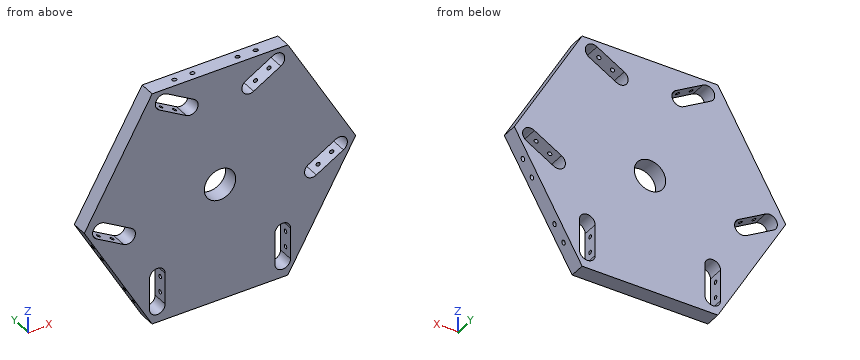
```python
from build123d import *

# Parameters (mm, degrees)
BOSS_EXTRUDE1_DEPTH     = 10
CUT_EXTRUDE1_DEPTH      = 20
SKETCH4_R               = 1.25
CUT_EXTRUDE2_DEPTH      = 149.417392118
CUT_EXTRUDE3_DEPTH      = 116
CUT_EXTRUDE3_DEPTH_BACK = 116
SKETCH6_R               = 10
CIRPATTERN1_COUNT       = 3


with BuildPart() as part:
    # Sketch1 → Boss-Extrude1 (new body)
    with BuildSketch(Plane(origin=(0, 0, 0), x_dir=(1, 0, 0), z_dir=(0, 1, 0))):
        Polygon((-43.301270189, -75), (43.301270189, -75), (86.602540378, 0), (43.301270189, 75), (-43.301270189, 75), (-86.602540378, 0), align=None)
    extrude(amount=BOSS_EXTRUDE1_DEPTH)

    # Sketch3 → Cut-Extrude1 (cut)
    with BuildSketch(Plane(origin=(0, 10, 0), x_dir=(1, 0, 0), z_dir=(0, 1, 0))):
        with BuildLine():
            Line((-78.791651246, 6.47114317), (-61.47114317, 16.47114317))
            ThreePointArc((-61.47114317, 16.47114317), (-54.641016151, 14.641016151), (-56.47114317, 7.810889132))
            Line((-56.47114317, 7.810889132), (-73.791651246, -2.189110868))
            ThreePointArc((-73.791651246, -2.189110868), (-80.621778265, -0.358983849), (-78.791651246, 6.47114317))
        make_face()
        with BuildLine():
            Line((-38.791651246, -62.810889132), (-21.47114317, -52.810889132))
            ThreePointArc((-21.47114317, -52.810889132), (-14.641016151, -54.641016151), (-16.47114317, -61.47114317))
            Line((-16.47114317, -61.47114317), (-33.791651246, -71.47114317))
            ThreePointArc((-33.791651246, -71.47114317), (-40.621778265, -69.641016151), (-38.791651246, -62.810889132))
        make_face()
    cut_extrude1 = extrude(amount=-CUT_EXTRUDE1_DEPTH, mode=Mode.SUBTRACT)

    # Sketch4 → Cut-Extrude2 (cut, symmetric)
    with BuildSketch(Plane(origin=(17.5, 0, 30.310889132), x_dir=(0.8660254037844383, 0, -0.5000000000000007), z_dir=(0.5000000000000007, 0, 0.8660254037844383))):
        with Locations((-60, 5)):
            Circle(SKETCH4_R)
        with Locations((-50, 5)):
            Circle(SKETCH4_R)
    cut_extrude2 = extrude(amount=CUT_EXTRUDE2_DEPTH, both=True, mode=Mode.SUBTRACT)

    # Sketch6 → Cut-Extrude3 (cut, two sides: drawn at the far end of the back side and taken through both)
    with BuildSketch(Plane(origin=(0, 10, 0), x_dir=(1, 0, 0), z_dir=(0, 1, 0)).offset(-CUT_EXTRUDE3_DEPTH_BACK)):
        with Locations(Location((0, 0, 0), (0, 0, 270))):
            Circle(SKETCH6_R)
    extrude(amount=CUT_EXTRUDE3_DEPTH + CUT_EXTRUDE3_DEPTH_BACK, mode=Mode.SUBTRACT)

    # CirPattern1: Cut-Extrude1, Cut-Extrude2 ×3 about axis
    cirpattern1_axis = Axis((0, 0, 0), (0, 1, 0))
    add([cut_extrude1.rotate(cirpattern1_axis, i * 360 / CIRPATTERN1_COUNT) for i in range(1, CIRPATTERN1_COUNT)], mode=Mode.SUBTRACT)
    add([cut_extrude2.rotate(cirpattern1_axis, i * 360 / CIRPATTERN1_COUNT) for i in range(1, CIRPATTERN1_COUNT)], mode=Mode.SUBTRACT)


solid = part.part
```
CAD build for the part. Positions are in the model's coordinates, mm. Round coordinates to 2 decimals unless told otherwise and drop trailing zeros. Order: outer loops, then holes, each group sorted by start corner. A loop starts at its lowest first (then second) coordinate and runs counter-clockwise, first axis right, second up. Notation, with made-up numbers: (51, 60) -> (110, 60) arc R23 ccw to (110, 71) -> close; hole circle Ø5 at (74, 44.25). An arc over 180 degrees is marked (long way). One line per question, with ' | ' between items.
Q1. Probe probe 1 along Y at (x, z) = (-49, -60); probe 2 along X at (y, z) = (9.5, -43.5); probe 3 along Z at (x, y) = (0, 5.5). List the from-to ranges inside material, lowest first.
Completed:
probe 1: y = 0 to 3.75, 6.25 to 10 | probe 2: x = -61.49 to -44.77, -35.23 to 35.23, 44.77 to 61.49 | probe 3: z = -75 to -61.15, -58.85 to -51.15, -48.85 to -10, 10 to 75
Q2. Slice it at A-A (x = 0). Write the cut outline in (y, z).
Completed:
outline: (0, -75) -> (10, -75) -> (10, -10) -> (0, -10) -> close; (0, 10) -> (10, 10) -> (10, 75) -> (0, 75) -> close; hole circle Ø2.5 at (5, -60); hole circle Ø2.5 at (5, -50)
Q3. Drop flat-ended pins along their axis: pin 1 (6 mm diameter, centred on y = 5.5, z = 43.5, fed in from +X); pin 2 (1 mm diameter, centred on x = -55.5, y = 3.5, fed in from +Z); pin 3 (5 mm diameter, centred on y = 5.5, z = -58.5, fed in from +X). Give the stop position or say it passes through.
Completed:
pin 1: stops at x = 63.22 | pin 2: stops at z = 54.74 | pin 3: stops at x = 54.27
Q4. Slice it at B-B (z = 31.5). Give the number of separate pieces and of enclosed holes in the cut face, then the cut area to 3 significant figures.
Completed:
separate pieces: 1 | enclosed holes: 4 | area: 1,350 mm^2
